from build123d import *

# Parameters (mm, degrees)
SKETCH1_W           = 20.6
SKETCH1_H           = 4
BOSS_EXTRUDE1_DEPTH = 18
SKETCH2_W           = 16
SKETCH2_H           = 18
BOSS_EXTRUDE3_DEPTH = 4
SKETCH3_W           = 20.6
SKETCH3_H           = 4
BOSS_EXTRUDE4_DEPTH = 12
SKETCH4_R           = 4.9
BOSS_EXTRUDE5_DEPTH = 5
SKETCH5_W           = 10
SKETCH5_H           = 6
CUT_EXTRUDE1_DEPTH  = 10
BOSS_EXTRUDE6_DEPTH = 4
CHAMFER1_SIZE       = 0.5
CHAMFER2_SIZE       = 0.5


with BuildPart() as part:
    # Sketch1 → Boss-Extrude1 (new body)
    with BuildSketch(Plane(origin=(0, 0, 0), x_dir=(1, 0, 0), z_dir=(0, 1, 0))):
        Rectangle(SKETCH1_W, SKETCH1_H)
    extrude(amount=BOSS_EXTRUDE1_DEPTH)

    # Sketch2 → Boss-Extrude3 (add)
    with BuildSketch(Plane.ZY.offset(10.3)):
        with Locations((6, 9)):
            Rectangle(SKETCH2_W, SKETCH2_H)
    boss_extrude3 = extrude(amount=BOSS_EXTRUDE3_DEPTH)

    # Mirror1: Boss-Extrude3 across plane
    add(boss_extrude3.mirror(Plane.ZY))

    # Sketch3 → Boss-Extrude4 (add)
    with BuildSketch(Plane.XY.offset(2)):
        with Locations((0, 2)):
            Rectangle(SKETCH3_W, SKETCH3_H)
    extrude(amount=BOSS_EXTRUDE4_DEPTH)

    # Sketch4 → Boss-Extrude5 (add)
    with BuildSketch(Plane(origin=(0, 0, -2), x_dir=(-1, 0, 0), z_dir=(0, 0, -1))):
        with Locations(Location((0, 14, 0), (0, 0, 125.281261827))):
            Circle(SKETCH4_R)
    extrude(amount=BOSS_EXTRUDE5_DEPTH)

    # Sketch5 → Cut-Extrude1 (cut)
    with BuildSketch(Plane(origin=(0, 4, 0), x_dir=(1, 0, 0), z_dir=(0, 1, 0))):
        with Locations((0, -8)):
            Rectangle(SKETCH5_W, SKETCH5_H)
    extrude(amount=-CUT_EXTRUDE1_DEPTH, mode=Mode.SUBTRACT)

    # Sketch6 → Boss-Extrude6 (add)
    with BuildSketch(Plane(origin=(0, 18, 0), x_dir=(1, 0, 0), z_dir=(0, 1, 0))):
        Polygon((-10.3, -2), (10.3, -2), (10.3, -14), (14.3, -14), (14.3, 2), (2.83019434, 2), (-2.83019434, 2), (-14.3, 2), (-14.3, -14), (-10.3, -14), align=None)
    extrude(amount=BOSS_EXTRUDE6_DEPTH)

    # Chamfer1
    chamfer1_edges = [part.edges().sort_by_distance(p)[0] for p in [
        (0, 0, 14),
        (-14.3, 11, -2),
        (-14.3, 0, 6),
        (14.3, 11, -2),
        (14.3, 11, 14),
        (14.3, 0, 6),
        (-10.3, 13, 14),
        (0, 4, 14),
        (-10.3, 4, 8),
        (0, 0, -2),
        (-2.83019434, 10, -2),
        (-2.83019434, 10, -7),
        (5, 0, 8),
        (0, 0, 11),
        (5, 2, 11),
        (-5, 0, 8),
        (-5, 2, 11),
        (0, 0, 5),
        (-5, 2, 5),
        (5, 4, 8),
        (0, 4, 5),
        (-5, 4, 8),
        (0, 4, 11),
        (-10.3, 13, 2),
        (-10.3, 22, 8),
        (0, 22, 2),
        (14.3, 22, 6),
        (0, 22, -2),
    ]]
    chamfer(chamfer1_edges, length=CHAMFER1_SIZE)

    # Chamfer2
    chamfer2_edges = [part.edges().sort_by_distance(p)[0] for p in [
        (5, 2, 5),
        (10.3, 4, 7.75),
        (-14.3, 22, 6.25),
        (-14.3, 11.25, 14),
        (10.3, 12.75, 2),
        (10.3, 12.75, 14),
        (0.25, 4, 2),
        (10.3, 22, 7.75),
        (12.05, 22, 14),
        (-12.55, 22, 14),
    ]]
    chamfer(chamfer2_edges, length=CHAMFER2_SIZE - 0.0001)  # a hair under: the kernel refuses the full size


solid = part.part
Design review of the part built by this model. Coordinates are the model's own, in mm. A direction names the side the tool comes from. Round coordinates to 2 decimals unless told otherwise and drop trailing zeros. Write each loop counter-clockwise with the first axis right and the second up, starting at its lowest first coordinate (ties: lowest second). Pieces come first, ordered by that corner, then holes. Notation, with made-up numbers: M -36.75,-28.75 L 15.25,-28.75 A9 cw 15.25,-13.75 Z; hole C 54,-35.75 d8. An arc over 180 degrees is marked long. One line per item, written item: value. Start each with the question number.
1. To check wall thickness, follow probe 1 along Z at (x, y) = (0.25, 1.5); probe 2 along X at (y, z) = (1, 8.5); probe 3 along Z at (x, y) = (0.75, 21.25). State the ranges of each line that lie inside material, in increasing order. Write a range as from..to.
2. Take a section at A-A on z = 7.75. State the section outline as (x, y) points.
3. For faces 1 (the face through (0, 4, 12)), 2 (the face through (-5, 2, 8)), 3 (the face through (1.08, 18.78, -4.47)), 4 (the face through (4.9, 3.8, 10.9)), list the 3-axis set-ups (+Z, -Z, +X, -X, +Y, -Y) from which the entire face can be reached by the end or side of a thin tool; tool diameter is ignored.
4. Take a section at D-D on z = 3.25. State the section outline as (x, y) points, then the cut area to 3 significant figures.
5. Clearance check with flat-ended pins moving along their axes: P1, Ø3, axis at x = 9, y = 7.5, coming from the -Z side; P2, Ø5, axis at x = -5, y = 14.5, coming from the +Z side; P3, Ø1, axis at x = 2.5, z = 9, coming from the +Y side. State where each tip first meets the part, or that it passes through.
6. Draft analysis for pull direction Z (two halves, no side actions). For faces 5 (the face through (4.9, 0.2, 10.9)), 6 (the face through (5, 2, 8)), 7 (the face through (0.4, 3.8, 13.7)), 8 (the face through (3, 9, -2)), state which applies: pulls with the +Z half, pulls with the -Z half, needs draft (parallel to the pull), parting line crosses it, or undercut.
7. Take a section at B-B on y = 6.75. State the section outline as (x, z) points.
8. Take a section at C-C on x = 0. State the section outline as (y, z) points.
Computed:
1. probe 1: z = -2..5, 11..14
1. probe 2: x = -14.3..-5, 5..14.3
1. probe 3: z = -2..2
2. outline: M -14.3,0.5 L -13.8,0 L -5.5,0 L -5,0.5 L -5,3.5 L -5.5,4 L -9.8,4 L -10.3,4.5 L -10.3,21.5 L -10.8,22 L -13.8,22 L -14.3,21.5 Z; M 5,0.5 L 5.5,0 L 13.8,0 L 14.3,0.5 L 14.3,21.5 L 13.8,22 L 10.8,22 L 10.3,21.5 L 10.3,4.5 L 9.8,4 L 5.5,4 L 5,3.5 Z
3. face 1: +Z, +Y
3. face 2: +Y, -Y
3. face 3: -Z
3. face 4: +Y
4. outline: M -14.3,0.5 L -13.8,0 L 13.8,0 L 14.3,0.5 L 14.3,21.5 L 13.8,22 L 10.8,22 L 10.3,21.5 L 10.3,4.5 L 9.8,4 L -9.8,4 L -10.3,4.5 L -10.3,21.5 L -10.8,22 L -13.8,22 L -14.3,21.5 Z
4. area: 258 mm²
5. P1: stops at z = -2
5. P2: stops at z = 2
5. P3: passes through
6. face 5: undercut
6. face 6: undercut
6. face 7: pulls with the +Z half
6. face 8: pulls with the -Z half
7. outline: M -14.3,-1.5 L -13.8,-2 L 13.8,-2 L 14.3,-1.5 L 14.3,13.5 L 13.8,14 L 10.8,14 L 10.3,13.5 L 10.3,2.5 L 9.8,2 L -9.8,2 L -10.3,2.5 L -10.3,13.5 L -10.8,14 L -13.8,14 L -14.3,13.5 Z
8. outline: M 0,-1.5 L 0.5,-2 L 8.6,-2 L 9.1,-2.5 L 9.1,-6.5 L 9.6,-7 L 18.4,-7 L 18.9,-6.5 L 18.9,-2.5 L 19.4,-2 L 21.5,-2 L 22,-1.5 L 22,1.5 L 21.5,2 L 4.5,2 L 4,2.5 L 4,4.5 L 3.5,5 L 0.5,5 L 0,4.5 Z; M 0,11.5 L 0.5,11 L 3.5,11 L 4,11.5 L 4,13.5 L 3.5,14 L 0.5,14 L 0,13.5 Z
